Could you check a few things on this drawing? It's one solid part, dimensions in mm from its lowest x, y, z. Coordinates: 2 decimals unless noted, no trailing zeros. Write each loop counter-clockwise with the first axis right and the second up, starting at its lowest first coordinate (ties: lowest second). Pieces come first, ordered by that corner, then holes.
Item 1: I want a section at A-A (x = 36). Please give me the cut outline in (y, z).
Item 2: I want a section at B-B (y = 1.05). Count the separate pieces of the cut face and the enclosed holes in it, and give its area (3 significant figures).
Item 3: Please list where these lines run through material, in increasing order: line 1 (X direction, y = 0.2, z = 35.5); line 2 (X direction, y = 1.6, z = 24.5); line 3 (Z direction, x = 48, y = 1.1).
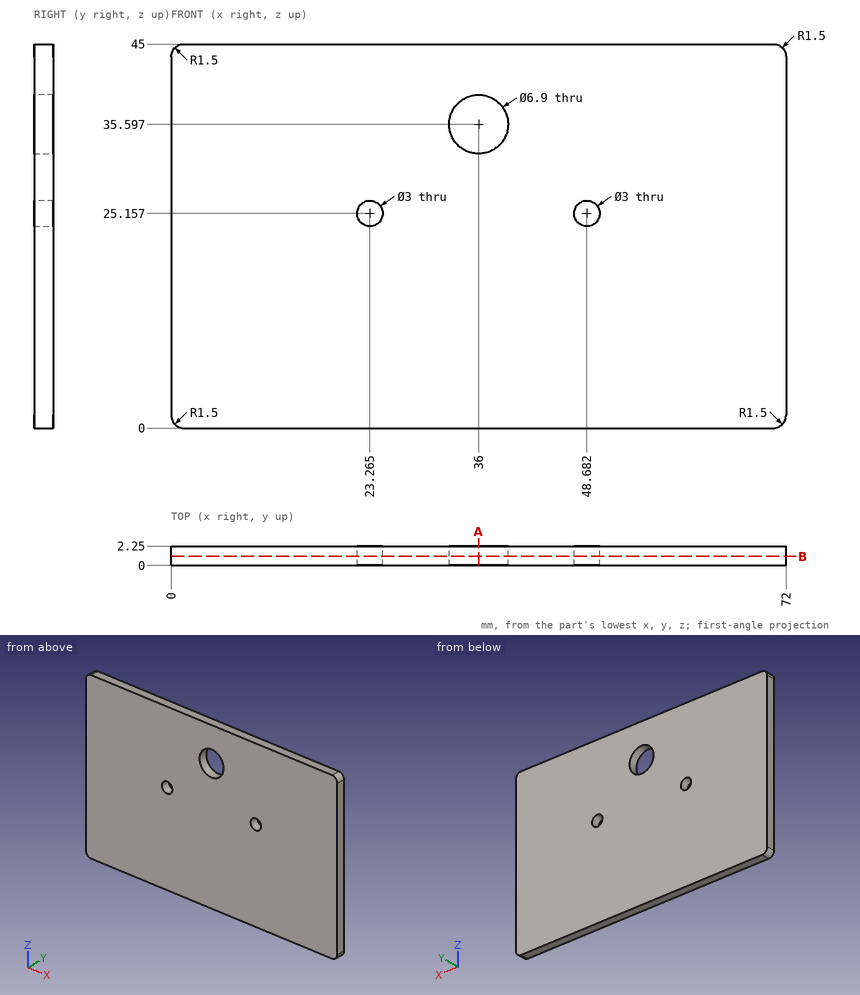
Answer:
1. outline: (0, 0) - (2.25, 0) - (2.25, 32.15) - (0, 32.15) - close; (0, 39.05) - (2.25, 39.05) - (2.25, 45) - (0, 45) - close
2. separate pieces: 1
2. enclosed holes: 3
2. area: 3,190 mm2
3. line 1: x = 0 to 32.55, 39.45 to 72
3. line 2: x = 0 to 21.92, 24.61 to 47.33, 50.03 to 72
3. line 3: z = 0 to 23.82, 26.49 to 45
